from build123d import *

# Parameters (mm, degrees)
BOSS_EXTRUDE1_DEPTH            = 29
SKETCH2_R                      = 2.6
SKETCH2_R_2                    = 1.55
BOSS_EXTRUDE3_DEPTH            = 5
CUT_EXTRUDE1_REACH             = 108.142
CUT_EXTRUDE1_DIRECTION_2_DEPTH = 107.141922264
CUT_EXTRUDE2_REACH             = 108.142
CUT_EXTRUDE2_DIRECTION_2_DEPTH = 107.141922264
FILLET1_R                      = 2
SKETCH6_R                      = 1.55
BOSS_EXTRUDE4_DEPTH            = 1


with BuildPart() as part:
    # Sketch1 → Boss-Extrude1 (new body)
    with BuildSketch(Plane(origin=(0, 0, 0), x_dir=(1, 0, 0), z_dir=(0, 1, 0))):
        Polygon((-13.5, 0), (0, 92.188031325), (13.5, 0), (14.489447114, 0.144894471), (0, 99.089605913), (-14.489447114, 0.144894471), align=None)
    extrude(amount=BOSS_EXTRUDE1_DEPTH)

    # Sketch2 → Boss-Extrude3 (add)
    # profile 1 of 10: a face of its own
    with BuildSketch(Plane(origin=(0, 0, 0), x_dir=(1, 0, 0), z_dir=(0, 1, 0))):
        with Locations((11.916884617, -0.231831154)):
            Circle(SKETCH2_R)
        with Locations(Location((11.916884617, -0.231831154, 0), (0, 0, 270))):
            Circle(SKETCH2_R_2, mode=Mode.SUBTRACT)
    # profile 2 of 10: a face of its own
    with BuildSketch(Plane(origin=(0, 0, 0), x_dir=(1, 0, 0), z_dir=(0, 1, 0))):
        with Locations((9.888362021, 13.620428448)):
            Circle(SKETCH2_R)
        with Locations(Location((9.888362021, 13.620428448, 0), (0, 0, 270))):
            Circle(SKETCH2_R_2, mode=Mode.SUBTRACT)
    # profile 3 of 10: a face of its own
    with BuildSketch(Plane(origin=(0, 0, 0), x_dir=(1, 0, 0), z_dir=(0, 1, 0))):
        with Locations((7.859839425, 27.47268805)):
            Circle(SKETCH2_R)
        with Locations(Location((7.859839425, 27.47268805, 0), (0, 0, 270))):
            Circle(SKETCH2_R_2, mode=Mode.SUBTRACT)
    # profile 4 of 10: a face of its own
    with BuildSketch(Plane(origin=(0, 0, 0), x_dir=(1, 0, 0), z_dir=(0, 1, 0))):
        with Locations((5.831316829, 41.324947652)):
            Circle(SKETCH2_R)
        with Locations(Location((5.831316829, 41.324947652, 0), (0, 0, 270))):
            Circle(SKETCH2_R_2, mode=Mode.SUBTRACT)
    # profile 5 of 10: a face of its own
    with BuildSketch(Plane(origin=(0, 0, 0), x_dir=(1, 0, 0), z_dir=(0, 1, 0))):
        with Locations((3.802794233, 55.177207254)):
            Circle(SKETCH2_R)
        with Locations(Location((3.802794233, 55.177207254, 0), (0, 0, 270))):
            Circle(SKETCH2_R_2, mode=Mode.SUBTRACT)
    # profile 6 of 10: a face of its own
    with BuildSketch(Plane(origin=(0, 0, 0), x_dir=(1, 0, 0), z_dir=(0, 1, 0))):
        with Locations((-11.916884617, -0.231831154)):
            Circle(SKETCH2_R)
        with Locations(Location((-11.916884617, -0.231831154, 0), (0, 0, 90))):
            Circle(SKETCH2_R_2, mode=Mode.SUBTRACT)
    # profile 7 of 10: a face of its own
    with BuildSketch(Plane(origin=(0, 0, 0), x_dir=(1, 0, 0), z_dir=(0, 1, 0))):
        with Locations((-9.888362021, 13.620428448)):
            Circle(SKETCH2_R)
        with Locations(Location((-9.888362021, 13.620428448, 0), (0, 0, 90))):
            Circle(SKETCH2_R_2, mode=Mode.SUBTRACT)
    # profile 8 of 10: a face of its own
    with BuildSketch(Plane(origin=(0, 0, 0), x_dir=(1, 0, 0), z_dir=(0, 1, 0))):
        with Locations((-7.859839425, 27.47268805)):
            Circle(SKETCH2_R)
        with Locations(Location((-7.859839425, 27.47268805, 0), (0, 0, 90))):
            Circle(SKETCH2_R_2, mode=Mode.SUBTRACT)
    # profile 9 of 10: a face of its own
    with BuildSketch(Plane(origin=(0, 0, 0), x_dir=(1, 0, 0), z_dir=(0, 1, 0))):
        with Locations((-5.831316829, 41.324947652)):
            Circle(SKETCH2_R)
        with Locations(Location((-5.831316829, 41.324947652, 0), (0, 0, 90))):
            Circle(SKETCH2_R_2, mode=Mode.SUBTRACT)
    # profile 10 of 10: a face of its own
    with BuildSketch(Plane(origin=(0, 0, 0), x_dir=(1, 0, 0), z_dir=(0, 1, 0))):
        with Locations((-3.802794233, 55.177207254)):
            Circle(SKETCH2_R)
        with Locations(Location((-3.802794233, 55.177207254, 0), (0, 0, 90))):
            Circle(SKETCH2_R_2, mode=Mode.SUBTRACT)
    boss_extrude3 = extrude(amount=BOSS_EXTRUDE3_DEPTH)

    # Cut-Extrude1: up to this face of the body (flat: up to its plane)
    cut_extrude1_end = Plane(part.part.faces().sort_by_distance((-6.671349584, 14.924053366, -46.631099147))[0])
    # Sketch4 → Cut-Extrude1 (cut, up to the picked face)
    with BuildSketch(Plane(origin=(0.283424505, 0, 1.935433121), x_dir=(0.9894471144188783, 0, -0.14489447114419254), z_dir=(0.14489447114419252, 0, 0.9894471144188782)), mode=Mode.PRIVATE) as cut_extrude1_sk1:
        Polygon((13.357536045, 5), (9.157536045, 5), (9.157536045, 1.475781549), align=None)
    cut_extrude1_tool1 = split(extrude(cut_extrude1_sk1.sketch, amount=-CUT_EXTRUDE1_REACH, mode=Mode.PRIVATE), bisect_by=cut_extrude1_end, keep=Keep.BOTH, mode=Mode.PRIVATE)
    cut_extrude1 = cut_extrude1_tool1.solids().sort_by(Axis((10.729548, 3.825261, 0.405705), (-0.14489447114419252, 0, -0.9894471144188782)))[0]
    add(cut_extrude1, mode=Mode.SUBTRACT)

    # Sketch4 → Cut-Extrude1 direction 2 (cut)
    with BuildSketch(Plane(origin=(0.283424505, 0, 1.935433121), x_dir=(0.9894471144188783, 0, -0.14489447114419254), z_dir=(0.14489447114419252, 0, 0.9894471144188782))):
        Polygon((13.357536045, 5), (9.157536045, 5), (9.157536045, 1.475781549), align=None)
    cut_extrude1_direction_2 = extrude(amount=CUT_EXTRUDE1_DIRECTION_2_DEPTH, mode=Mode.SUBTRACT)

    # Cut-Extrude2: up to this face of the body (flat: up to its plane)
    cut_extrude2_end = Plane(part.part.faces().sort_by_distance((6.671349584, 14.924053366, -46.631099147))[0])
    # Sketch5 → Cut-Extrude2 (cut, up to the picked face)
    with BuildSketch(Plane(origin=(-0.283424505, 0, 1.935433121), x_dir=(0.9894471144188784, 0, 0.14489447114419146), z_dir=(-0.14489447114419146, 0, 0.9894471144188784)), mode=Mode.PRIVATE) as cut_extrude2_sk1:
        Polygon((-9.157536045, 5), (-9.157536045, 1.475781549), (-13.357536045, 5), align=None)
    cut_extrude2_tool1 = split(extrude(cut_extrude2_sk1.sketch, amount=-CUT_EXTRUDE2_REACH, mode=Mode.PRIVATE), bisect_by=cut_extrude2_end, keep=Keep.BOTH, mode=Mode.PRIVATE)
    cut_extrude2 = cut_extrude2_tool1.solids().sort_by(Axis((-10.729548, 3.825261, 0.405705), (0.14489447114419146, 0, -0.9894471144188784)))[0]
    add(cut_extrude2, mode=Mode.SUBTRACT)

    # Sketch5 → Cut-Extrude2 direction 2 (cut)
    with BuildSketch(Plane(origin=(-0.283424505, 0, 1.935433121), x_dir=(0.9894471144188784, 0, 0.14489447114419146), z_dir=(-0.14489447114419146, 0, 0.9894471144188784))):
        Polygon((-9.157536045, 5), (-9.157536045, 1.475781549), (-13.357536045, 5), align=None)
    cut_extrude2_direction_2 = extrude(amount=CUT_EXTRUDE2_DIRECTION_2_DEPTH, mode=Mode.SUBTRACT)

    # Mirror2: Boss-Extrude3, Cut-Extrude1, Cut-Extrude1 direction 2, Cut-Extrude2, Cut-Extrude2 direction 2 across plane
    add(boss_extrude3.mirror(Plane.ZX.offset(14.5)))
    add(cut_extrude1.mirror(Plane.ZX.offset(14.5)), mode=Mode.SUBTRACT)
    add(cut_extrude1_direction_2.mirror(Plane.ZX.offset(14.5)), mode=Mode.SUBTRACT)
    add(cut_extrude2.mirror(Plane.ZX.offset(14.5)), mode=Mode.SUBTRACT)
    add(cut_extrude2_direction_2.mirror(Plane.ZX.offset(14.5)), mode=Mode.SUBTRACT)

    # Fillet1
    # the kernel refuses this fillet: 2 mm, written as the material it adds along each edge
    with BuildSketch(Plane(origin=(13.5, 5, 0), x_dir=(0, 1, 0), z_dir=(0.9894471144188783, 0, -0.1448944711441925))) as fillet1_piece_1_section:
        with BuildLine():
            CenterArc((FILLET1_R, FILLET1_R), FILLET1_R, 180, 90)
            Line((0, FILLET1_R), (0, 0))
            Line((0, 0), (FILLET1_R, 0))
        make_face()
    fillet1_piece_1 = extrude(amount=6, mode=Mode.PRIVATE)
    fillet1_piece_1 = fillet1_piece_1 & Plane(origin=(11.916884617, 5.699977741, 0.231831154), x_dir=(1, 0, 0), z_dir=(0, -1, 0)) * Cylinder(2.6, 20, mode=Mode.PRIVATE)
    add(fillet1_piece_1)
    with BuildSketch(Plane(origin=(13.5, 24, 0), x_dir=(0, -1, 0), z_dir=(0.9894471144188783, 0, -0.1448944711441925))) as fillet1_piece_2_section:
        with BuildLine():
            CenterArc((FILLET1_R, -FILLET1_R), FILLET1_R, 90, 90)
            Line((0, -FILLET1_R), (0, 0))
            Line((0, 0), (FILLET1_R, 0))
        make_face()
    fillet1_piece_2 = extrude(amount=6, mode=Mode.PRIVATE)
    fillet1_piece_2 = fillet1_piece_2 & Plane(origin=(11.916884617, 23.30002226, 0.231831154), x_dir=(1, 0, 0), z_dir=(0, 1, 0)) * Cylinder(2.6, 20, mode=Mode.PRIVATE)
    add(fillet1_piece_2)
    with BuildSketch(Plane(origin=(-19.436682687, 24, -0.869366827), x_dir=(0, -1, 0), z_dir=(0.9894471144188784, 0, 0.1448944711441914))) as fillet1_piece_3_section:
        with BuildLine():
            CenterArc((FILLET1_R, -FILLET1_R), FILLET1_R, 90, 90)
            Line((0, -FILLET1_R), (0, 0))
            Line((0, 0), (FILLET1_R, 0))
        make_face()
    fillet1_piece_3 = extrude(amount=6, mode=Mode.PRIVATE)
    fillet1_piece_3 = fillet1_piece_3 & Plane(origin=(-11.916884617, 23.777637105, 0.231831154), x_dir=(1, 0, 0), z_dir=(0, 1, 0)) * Cylinder(2.6, 21, mode=Mode.PRIVATE)
    add(fillet1_piece_3)
    with BuildSketch(Plane(origin=(-19.436682687, 5, -0.869366827), x_dir=(-0.1448944711441914, 0, 0.9894471144188784), z_dir=(0.9894471144188784, 0, 0.1448944711441914))) as fillet1_piece_4_section:
        with BuildLine():
            CenterArc((FILLET1_R, -FILLET1_R), FILLET1_R, 90, 90)
            Line((0, -FILLET1_R), (0, 0))
            Line((0, 0), (FILLET1_R, 0))
        make_face()
    fillet1_piece_4 = extrude(amount=6, mode=Mode.PRIVATE)
    fillet1_piece_4 = fillet1_piece_4 & Plane(origin=(-11.916884617, 5.222362792, 0.231831154), x_dir=(1, 0, 0), z_dir=(0, -1, 0)) * Cylinder(2.6, 21, mode=Mode.PRIVATE)
    add(fillet1_piece_4)

    # Sketch6 → Boss-Extrude4 (add)
    with BuildSketch(Plane.XZ):
        with Locations(Location((3.802794233, -55.177207254, 0), (0, 0, 270))):
            Circle(SKETCH6_R)
        with Locations(Location((-3.802794233, -55.177207254, 0), (0, 0, 270))):
            Circle(SKETCH6_R)
        with Locations(Location((-5.831316829, -41.324947652, 0), (0, 0, 270))):
            Circle(SKETCH6_R)
        with Locations(Location((5.831316829, -41.324947652, 0), (0, 0, 270))):
            Circle(SKETCH6_R)
        with Locations(Location((7.859839425, -27.47268805, 0), (0, 0, 270))):
            Circle(SKETCH6_R)
        with Locations(Location((-7.859839425, -27.47268805, 0), (0, 0, 270))):
            Circle(SKETCH6_R)
        with Locations(Location((-9.888362021, -13.620428448, 0), (0, 0, 270))):
            Circle(SKETCH6_R)
        with Locations(Location((9.888362021, -13.620428448, 0), (0, 0, 270))):
            Circle(SKETCH6_R)
        with Locations(Location((11.916884617, 0.231831154, 0), (0, 0, 270))):
            Circle(SKETCH6_R)
        with Locations(Location((-11.916884617, 0.231831154, 0), (0, 0, 270))):
            Circle(SKETCH6_R)
    extrude(amount=-BOSS_EXTRUDE4_DEPTH)


solid = part.part
Can you work these out from the model? Positions are in its coordinate system, mm. A direction names the side the tool comes from. Give positions to 0.01 mm unless a question says otherwise; leave off trailing zeros. Order: outer loops, then holes, each group sorted by start corner. A loop starts at its lowest first (then second) coordinate and runs counter-clockwise, first axis right, second up. Notation, with made-up numbers: M 78.5,46 L 118.5,46 A35 ccw 118.5,79 Z; hole C 34,33 d3. An arc over 180 degrees is marked long. Use one line per item in the form item = value.
Item 1: Thinking about a two-plate mould opening in Z: for faces 1 (the flat face through (-4, 0, -40)), 2 (the flat face through (-6.25, 26.57, -28.37)), 3 (the cylindrical face through (13.454, 27.107, 0.03)), which applies, pulls with the +Z half, pulls with the -Z half, needs draft (parallel to the pull), parting line crosses it, or undercut?
Values follow:
face_1 = needs draft
face_2 = pulls with the +Z half
face_3 = undercut
Item 2: Will these pins go through, and if not, where does the flat tip stop? pin 1 Ø3.5 at (x, z) = (-11.5, -0.5) entering from +Y; pin 2 Ø0.9 at (x, z) = (-9.5, -13.5) entering from +Y; pin 3 Ø12 at (y, z) = (5.5, -43.5) entering from +X; pin 4 Ø12 at (y, z) = (11.5, -14.5) entering from -X.
Values follow:
pin_1 = 29
pin_2 = 1
pin_3 = 9.02
pin_4 = -13.27
Item 3: For faces 4 (the flat face through (2.193, 26.57, -56.073)), 5 (the cylindrical face through (13.93, 23.13, 0.29)), 6 (the cylindrical face through (-13.946, 5.835, 0.313)), 7 (the flat face through (4, 1, -55)), which set-ups out of +Z, -Z, +X, -X, +Y, -Y let a thin tool reach every point of the face, with its end or its side?
Values follow:
face_4 = +Z
face_5 = +Z, +X
face_6 = +Z, -X
face_7 = +Y
Item 4: If we section it at B-B, the plane y = 16.5: Write out the boundary of the cut face in (x, z), and give its area (3 significant figures).
Values follow:
outline = M -14.49,-0.14 L 0,-99.09 L 14.49,-0.14 L 13.5,0 L 0,-92.19 L -13.5,0 Z
area = 193 mm^2
Item 5: If I drill on line 1 along X through (y, z) = (1.25, -26.5); line 2 along X through (y, z) = (27, -41.5); line 3 along X through (y, z) = (4.75, -24), over which ranges is the centre line in solid material (lowest first)? Write a range as [from, to].
Values follow:
line_1 = [-10.63, -9.07], [-6.65, -5.45], [5.45, 6.65], [9.07, 10.63]
line_2 = [-8.43, -7.37], [-4.29, -3.81], [3.81, 4.29], [7.37, 8.43]
line_3 = [-11, -9.99], [9.99, 11]
Item 6: If we section it at A-A, the plane z = -51: Write out the boundary of the cut face in (x, y), and give its area (3 significant figures).
Values follow:
outline = M -7.04,0 L -6.03,0 L -6.03,29 L -7.04,29 Z; M 6.03,0 L 7.04,0 L 7.04,29 L 6.03,29 Z
area = 58.6 mm^2
